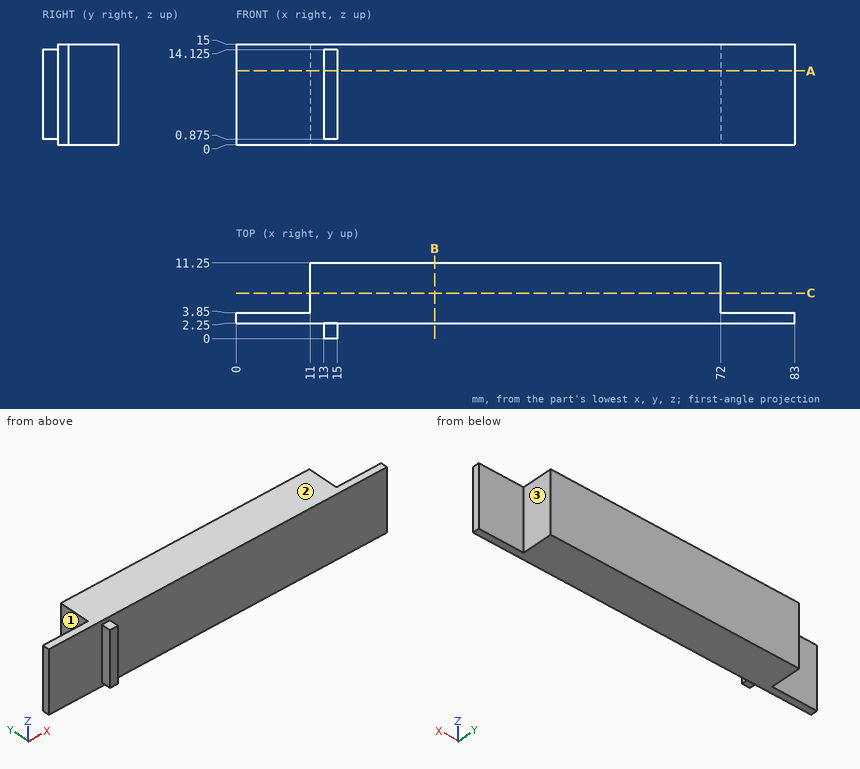
Source: three-view drawing plus pictorial views. Frame: mm from the lowest corner of the part. A direction names the side the tool comes from. Coordinates: 2 decimals unless noted, no trailing zeros. Loops run counter-clockwise (first coordinate to the right, second up) from the corner with the lowest first, then second, coordinate; pieces in that order, holes last. Notation, with made-up numbers: (-20, 57) - (-8, 57) arc R21 cw to (-8, 62) - close; hole circle Ø5 at (8, 77.5). An arc over 180 degrees is marked (long way). One line per item, written item: value. Start each with the question number.
1. Contact query for flat-ended pins moving along their axis: P1, Ø5, axis at x = 25, y = 9.5, coming from the -Z side; P2, Ø1.5, axis at y = 6, z = 4.5, coming from the +X side; P3, Ø1.8, axis at y = 1, z = 7, coming from the +X side; P4, Ø0.6, axis at x = 14.5, y = 0.5, coming from the -Z side (3 decimals). Output: stop coordinate, or through.
2. Section C-C (y = 6.75). Return the cut outline in (x, z), and give its area (3 significant figures).
3. Set-up query: the marked faces 1, 2 and 3. Return all of +Z, -Z, +X, -X, +Y, -Y with unobstructed straight access to the full face (end or side cutting, diameter ignored); none if empty.
4. Section A-A (z = 11). Return the cut outline in (x, y).
5. Section B-B (x = 29.5). Return the cut outline in (y, z).
6. Ray query, L1, parallel to Y at x = 17.5, z = 6; L2, parallel to X at y = 1.75, z = 10.75; L3, parallel to Y at x = 6, z = 4. Return the intervals inside material, ascending.
Verdict:
1. P1: stops at z = 0
1. P2: stops at x = 72
1. P3: stops at x = 15
1. P4: stops at z = 0.875
2. outline: (11, 0) - (72, 0) - (72, 15) - (11, 15) - close
2. area: 915 mm2
3. face 1: +Z, -Z, -X, +Y
3. face 2: +Z, +X, -X, +Y, -Y
3. face 3: +Z, -Z, +X, +Y
4. outline: (0, 2.25) - (13, 2.25) - (13, 0) - (15, 0) - (15, 2.25) - (83, 2.25) - (83, 3.85) - (72, 3.85) - (72, 11.25) - (11, 11.25) - (11, 3.85) - (0, 3.85) - close
5. outline: (2.25, 0) - (11.25, 0) - (11.25, 15) - (2.25, 15) - close
6. L1: y = 2.25 to 11.25
6. L2: x = 13 to 15
6. L3: y = 2.25 to 3.85
